The model under review builds one solid part; all positions refer to its coordinate system, in mm. Face numbers are marked on the shaded views. Give positions to 0.01 mm unless a question says otherwise; leave off trailing zeros. Order: outer loops, then holes, each group sorted by start corner. A loop starts at its lowest first (then second) coordinate and runs counter-clockwise, first axis right, second up. Notation, with made-up numbers: (57, -1.75) -> (116, -1.75) arc R18 ccw to (116, 12.25) -> close; hole circle Ø5 at (55, 84.25). An arc over 180 degrees is marked (long way). Answer as a JSON object with one key per item and string values. Group by question number.
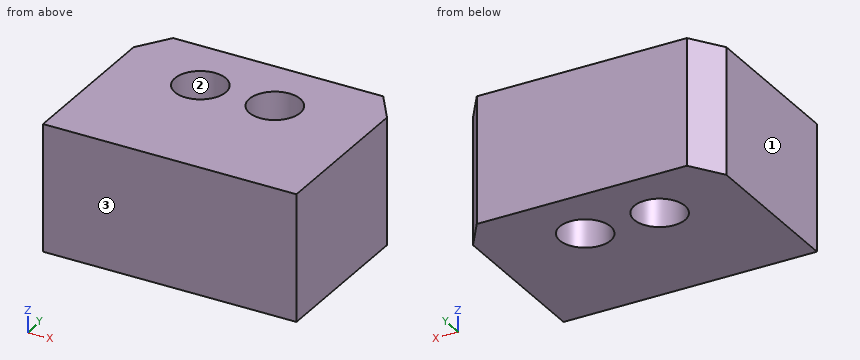
from build123d import *

# Parameters (mm, degrees)
ESBO_O1_R                = 4.020297227
RESSALTO_EXTRUS_O1_DEPTH = 20
ESBO_O2_W                = 40
ESBO_O2_H                = 20
RESSALTO_EXTRUS_O2_DEPTH = 10


with BuildPart() as part:
    # Esboço1 → Ressalto-extrusão1 (new body)
    with BuildSketch(Plane.XY):
        Polygon((19.906301529, -10.222394025), (-20.093698471, -10.222394025), (-20.093698471, 4.777605975), (-16.677218189, 9.709914003), (16.489821246, 9.709914003), (19.906301529, 4.777605975), align=None)
        with Locations((-6.819904998, 0)):
            Circle(ESBO_O1_R, mode=Mode.SUBTRACT)
        with Locations((4.930095002, 0)):
            Circle(ESBO_O1_R, mode=Mode.SUBTRACT)
    extrude(amount=RESSALTO_EXTRUS_O1_DEPTH)

    # Esboço2 → Ressalto-extrusão2 (add)
    with BuildSketch(Plane.XZ.offset(10.222394025)):
        with Locations((-0.093698471, 10)):
            Rectangle(ESBO_O2_W, ESBO_O2_H)
    extrude(amount=RESSALTO_EXTRUS_O2_DEPTH)


solid = part.part
1. Take a section at D-D on x = 4.5. Give the boundary of the cut face in (y, z), plus the area to 3 significant figures.
2. Take a section at A-A on y = 0. Give the boundary of the cut face in (x, z).
3. Take a section at B-B on z = 12. Give the boundary of the cut face in (x, y).
4. For probe 1 along Y at (x, z) = (5, 14.5); probe 2 along X at (y, z) = (1.5, 8.5); probe 3 along Y at (x, z) = (-9.5, 12.75), list the stretches that pass through material, from the lowest coordinate up. Write a range as [from, to].
5. Take a section at C-C on x = -7. Give the boundary of the cut face in (y, z), plus the area to 3 significant figures.
6. For pin 1 (6.5 mm diameter, centred on x = -6.82, y = 0, fed in from +Z), flat-tipped, find the tip position at first contact; note if it passes through.
7. Draft analysis for pull direction X (two halves, no side actions). For the marked faces 1, 2 and 3, state which applies: pulls with the +X half, pulls with the -X half, needs draft (parallel to the pull), parting line crosses it, or undercut.
Checks:
{
 "1": {"outline": "(-20.22, 0) -> (-4, 0) -> (-4, 20) -> (-20.22, 20) -> close; (4, 0) -> (9.71, 0) -> (9.71, 20) -> (4, 20) -> close", "area": "439 mm2"},
 "2": {"outline": "(-20.09, 0) -> (-10.84, 0) -> (-10.84, 20) -> (-20.09, 20) -> close; (-2.8, 0) -> (0.91, 0) -> (0.91, 20) -> (-2.8, 20) -> close; (8.95, 0) -> (19.91, 0) -> (19.91, 20) -> (8.95, 20) -> close"},
 "3": {"outline": "(-20.09, -20.22) -> (19.91, -20.22) -> (19.91, 4.78) -> (16.49, 9.71) -> (-16.68, 9.71) -> (-20.09, 4.78) -> close; hole circle Ø8.04 at (-6.82, 0); hole circle Ø8.04 at (4.93, 0)"},
 "4": {"probe 1": "y = [-20.22, -4.02], [4.02, 9.71]", "probe 2": "x = [-20.09, -10.55], [-3.09, 1.2], [8.66, 19.91]", "probe 3": "y = [-20.22, -3], [3, 9.71]"},
 "5": {"outline": "(-20.22, 0) -> (-4.02, 0) -> (-4.02, 20) -> (-20.22, 20) -> close; (4.02, 0) -> (9.71, 0) -> (9.71, 20) -> (4.02, 20) -> close", "area": "438 mm2"},
 "6": {"pin 1": "passes through"},
 "7": {"face 1": "pulls with the -X half", "face 2": "undercut", "face 3": "needs draft"}
}
